from build123d import *

# Parameters (mm, degrees)
F0_W     = 273.05
F0_H     = 228.6
F1_DEPTH = 19.05
F3_DEPTH = 19.05


with BuildPart() as f1:
    # F0 (on Right) → F1 (new body)
    with BuildSketch(Plane.YZ):
        with Locations((136.525, 114.3)):
            Rectangle(F0_W, F0_H)
    extrude(amount=-F1_DEPTH)

    # F2 (on face) → F3 (cut, through all)
    with BuildSketch(Plane.YZ):
        Polygon((182.033333, 139.7), (273.05, 139.7), (273.05, 228.6), (0, 228.6), (0, 0), (91.016667, 0), (91.016667, 69.85), (182.033333, 69.85), align=None)
    extrude(amount=-F3_DEPTH, mode=Mode.SUBTRACT)


solid = f1.part
Read the model definition and answer for the solid it produces. Units are mm, in the model's axes. A direction names the side the tool comes from. Round coordinates to 2 decimals unless told otherwise and drop trailing zeros. Order: outer loops, then holes, each group sorted by start corner. A loop starts at its lowest first (then second) coordinate and runs counter-clockwise, first axis right, second up. Notation, with made-up numbers: (-40, -6) - (10, -6) arc R7 cw to (10, -2) - close; hole circle Ø2 at (35, -32.75). An arc over 180 degrees is marked (long way). Use one line per item in the form item = value. Start each with the question number.
(1) The part is cut by section C-C (y = 156). Give the vertices of the cut face in (x, z), then the cut area to 3 significant figures.
(2) Determine the mould class of faces 3 (the face through (-19.05, 201, 55)), 4 (the face through (-9, 227, 139.7)), 5 (the face through (0, 201, 55)) for opening direction X: +X half, -X half, draft (parallel to the pull), parting line (faces both ways), or undercut.
(3) For faces 1 (the face through (-9, 136, 69.85)), 2 (the face through (-9, 91.017, 34)), determine the directions among +Z, -Z, +X, -X, +Y, -Y from which every point of the face is accessible in a straight line to the end or side of a thin tool.
(4) Find the intervals of material crossed by line 1 along Z through (x, y) = (-2.75, 119.5); line 2 along Y through (x, z) = (-11.5, 84), in increasing order. Write a range as from..to.
(5) The part is cut by section A-A (x = -11.75). Give the vertices of the cut face in (y, z), then the cut area to 3 significant figures.
(6) The part is cut by section B-B (z = 125). Give the vertices of the cut face in (x, y), then the cut area to 3 significant figures.
(7) Flat-ended cylindrical pins translate along their axes: pin 1 Ø5.5 at (x, z) = (-13, 89.5) entering from -Y; pin 2 Ø1.5 at (x, y) = (-5.5, 153) entering from +Z. Find the tip coordinate at first contact, or state that the pin passes through.
Checked values:
q1.outline = (-19.05, 0) - (0, 0) - (0, 69.85) - (-19.05, 69.85) - close
q1.area = 1,330 mm^2
q2.face_3 = -X half
q2.face_4 = draft
q2.face_5 = +X half
q3.face_1 = +Z, +X, -X, -Y
q3.face_2 = +Z, -Z, +X, -X, -Y
q4.line_1 = 0..69.85
q4.line_2 = 182.03..273.05
q5.outline = (91.02, 0) - (273.05, 0) - (273.05, 139.7) - (182.03, 139.7) - (182.03, 69.85) - (91.02, 69.85) - close
q5.area = 19,100 mm^2
q6.outline = (-19.05, 182.03) - (0, 182.03) - (0, 273.05) - (-19.05, 273.05) - close
q6.area = 1,730 mm^2
q7.pin_1 = 182.03
q7.pin_2 = 69.85
